from build123d import *

# Parameters (mm, degrees)
SKETCH1_R           = 2.1
SKETCH1_R_2         = 3.4
BOSS_EXTRUDE1_DEPTH = 160


with BuildPart() as part:
    # Sketch1 → Boss-Extrude1 (new body)
    with BuildSketch(Plane(origin=(0, 0, 0), x_dir=(0, 0, -1), z_dir=(1, 0, 0))):
        with BuildLine():
            Line((-15, 28), (-15, 19))
            Line((-15, 19), (-13, 19))
            Line((-13, 19), (-13, 23.25))
            Line((-13, 23.25), (-9.664213562, 23.25))
            Line((-9.664213562, 23.25), (-6, 19.585786438))
            Line((-6, 19.585786438), (-6, 10.414213562))
            Line((-6, 10.414213562), (-9.664213562, 6.75))
            Line((-9.664213562, 6.75), (-13, 6.75))
            Line((-13, 6.75), (-13, 11))
            Line((-13, 11), (-15, 11))
            Line((-15, 11), (-15, -11))
            Line((-15, -11), (-13, -11))
            Line((-13, -11), (-13, -6.75))
            Line((-13, -6.75), (-9.664213562, -6.75))
            Line((-9.664213562, -6.75), (-6, -10.414213562))
            Line((-6, -10.414213562), (-6, -19.585786438))
            Line((-6, -19.585786438), (-9.664213562, -23.25))
            Line((-9.664213562, -23.25), (-13, -23.25))
            Line((-13, -23.25), (-13, -19))
            Line((-13, -19), (-15, -19))
            Line((-15, -19), (-15, -28))
            ThreePointArc((-15, -28), (-14.414213562, -29.414213562), (-13, -30))
            Line((-13, -30), (-4, -30))
            Line((-4, -30), (-4, -28))
            Line((-4, -28), (-8.25, -28))
            Line((-8.25, -28), (-8.25, -24.664213562))
            Line((-8.25, -24.664213562), (-4.585786438, -21))
            Line((-4.585786438, -21), (4.585786438, -21))
            Line((4.585786438, -21), (8.25, -24.664213562))
            Line((8.25, -24.664213562), (8.25, -28))
            Line((8.25, -28), (4, -28))
            Line((4, -28), (4, -30))
            Line((4, -30), (13, -30))
            ThreePointArc((13, -30), (14.414213562, -29.414213562), (15, -28))
            Line((15, -28), (15, -19))
            Line((15, -19), (13, -19))
            Line((13, -19), (13, -23.25))
            Line((13, -23.25), (9.664213562, -23.25))
            Line((9.664213562, -23.25), (6, -19.585786438))
            Line((6, -19.585786438), (6, -10.414213562))
            Line((6, -10.414213562), (9.664213562, -6.75))
            Line((9.664213562, -6.75), (13, -6.75))
            Line((13, -6.75), (13, -11))
            Line((13, -11), (15, -11))
            Line((15, -11), (15, 11))
            Line((15, 11), (13, 11))
            Line((13, 11), (13, 6.75))
            Line((13, 6.75), (9.664213562, 6.75))
            Line((9.664213562, 6.75), (6, 10.414213562))
            Line((6, 10.414213562), (6, 19.585786438))
            Line((6, 19.585786438), (9.664213562, 23.25))
            Line((9.664213562, 23.25), (13, 23.25))
            Line((13, 23.25), (13, 19))
            Line((13, 19), (15, 19))
            Line((15, 19), (15, 28))
            ThreePointArc((15, 28), (14.414213562, 29.414213562), (13, 30))
            Line((13, 30), (4, 30))
            Line((4, 30), (4, 28))
            Line((4, 28), (8.25, 28))
            Line((8.25, 28), (8.25, 24.664213562))
            Line((8.25, 24.664213562), (4.585786438, 21))
            Line((4.585786438, 21), (-4.585786438, 21))
            Line((-4.585786438, 21), (-8.25, 24.664213562))
            Line((-8.25, 24.664213562), (-8.25, 28))
            Line((-8.25, 28), (-4, 28))
            Line((-4, 28), (-4, 30))
            Line((-4, 30), (-13, 30))
            ThreePointArc((-13, 30), (-14.414213562, 29.414213562), (-15, 28))
        make_face()
        with Locations((-11.6, 26.625)):
            Circle(SKETCH1_R, mode=Mode.SUBTRACT)
        with Locations((0, 15)):
            Circle(SKETCH1_R_2, mode=Mode.SUBTRACT)
        with Locations((11.6, 26.625)):
            Circle(SKETCH1_R, mode=Mode.SUBTRACT)
        with Locations((0, -15)):
            Circle(SKETCH1_R_2, mode=Mode.SUBTRACT)
        with Locations((-11.6, -26.625)):
            Circle(SKETCH1_R, mode=Mode.SUBTRACT)
        with Locations((11.6, -26.625)):
            Circle(SKETCH1_R, mode=Mode.SUBTRACT)
        with BuildLine():
            Line((-8.835786438, 4.75), (-12, 4.75))
            ThreePointArc((-12, 4.75), (-12.707106781, 4.457106781), (-13, 3.75))
            Line((-13, 3.75), (-13, -3.75))
            ThreePointArc((-13, -3.75), (-12.707106781, -4.457106781), (-12, -4.75))
            Line((-12, -4.75), (-8.835786438, -4.75))
            Line((-8.835786438, -4.75), (-3.651792162, -9.933994275))
            ThreePointArc((-3.651792162, -9.933994275), (-3.470780401, -10.020243756), (-3.275866789, -9.973202134))
            ThreePointArc((-3.275866789, -9.973202134), (0, -9), (3.275866789, -9.973202134))
            ThreePointArc((3.275866789, -9.973202134), (3.470780401, -10.020243756), (3.651792162, -9.933994275))
            Line((3.651792162, -9.933994275), (8.835786438, -4.75))
            Line((8.835786438, -4.75), (12, -4.75))
            ThreePointArc((12, -4.75), (12.707106781, -4.457106781), (13, -3.75))
            Line((13, -3.75), (13, 3.75))
            ThreePointArc((13, 3.75), (12.707106781, 4.457106781), (12, 4.75))
            Line((12, 4.75), (8.835786438, 4.75))
            Line((8.835786438, 4.75), (3.651792162, 9.933994275))
            ThreePointArc((3.651792162, 9.933994275), (3.470780401, 10.020243756), (3.275866789, 9.973202134))
            ThreePointArc((3.275866789, 9.973202134), (0, 9), (-3.275866789, 9.973202134))
            ThreePointArc((-3.275866789, 9.973202134), (-3.470780401, 10.020243756), (-3.651792162, 9.933994275))
            Line((-3.651792162, 9.933994275), (-8.835786438, 4.75))
        make_face(mode=Mode.SUBTRACT)
    extrude(amount=BOSS_EXTRUDE1_DEPTH)


solid = part.part
Design review of the part built by this model. Coordinates are the model's own, in mm. Give positions to 0.01 mm unless a question says otherwise; leave off trailing zeros. Loops run counter-clockwise (first coordinate to the right, second up) from the corner with the lowest first, then second, coordinate; pieces in that order, holes last. Notation, with made-up numbers: (75.25, 86.5) - (112.25, 86.5) arc R10 ccw to (112.25, 104.5) - close; hole circle Ø4 at (87.5, 61.5). An arc over 180 degrees is marked (long way). Write item = value, one per line.
1) Take a section at D-D on x = 79.5. Count the separate pieces of the cut face and the enclosed holes in it, and give its area (4 significant figures).
Result sheet:
separate_pieces = 1
enclosed_holes = 7
area = 592.5 mm2
2) Take a section at A-A on y = 2. State the section outline as (x, z) points, and give its area (3 significant figures).
Result sheet:
outline = (0, -15) - (160, -15) - (160, -13) - (0, -13) - close; (0, 13) - (160, 13) - (160, 15) - (0, 15) - close
area = 640 mm2
3) Take a section at B-B on z = 0. State the section outline as (x, y) points, and give its area (3 significant figures).
Result sheet:
outline = (0, -21) - (160, -21) - (160, -18.4) - (0, -18.4) - close; (0, -11.6) - (160, -11.6) - (160, -9) - (0, -9) - close; (0, 9) - (160, 9) - (160, 11.6) - (0, 11.6) - close; (0, 18.4) - (160, 18.4) - (160, 21) - (0, 21) - close
area = 1,660 mm2
4) Take a section at C-C on y = -15. State the section outline as (x, z) points, and give its area (3 significant figures).
Result sheet:
outline = (0, -6) - (160, -6) - (160, -3.4) - (0, -3.4) - close; (0, 3.4) - (160, 3.4) - (160, 6) - (0, 6) - close
area = 832 mm2
5) Draft analysis for pull direction Y (two halves, no side actions). For faces 1 (the face through (79, -28, -6)), 2 (the face through (79, -30, -8)), 3 (the face through (79, -24, -15)), state which applies: +Y half, -Y half, draft (parallel to the pull), parting line (faces both ways), or undercut.
Result sheet:
face_1 = undercut
face_2 = -Y half
face_3 = draft
6) To check wall thickness, follow line 1 (Y direction, x = 84, z = 0); line 2 (Y direction, x = 122, z = -11.6) (3 decimals); line 3 (Z direction, x = 68.5, y = 1.5). State the ranges of each line that lie inside material, in increasing order.
Result sheet:
line_1 = -21 to -18.4, -11.6 to -9, 9 to 11.6, 18.4 to 21
line_2 = -30 to -28.725, -24.525 to -23.25, -6.75 to -4.75, 4.75 to 6.75, 23.25 to 24.525, 28.725 to 30
line_3 = -15 to -13, 13 to 15
7) Clearance check with flat-ended pins moving along their axes: pin 1 Ø2 at (x, z) = (71, 14) entering from +Y; pin 2 Ø2 at (x, y) = (113, 29.5) entering from -Z; pin 3 Ø3 at (x, y) = (119.5, 13.5) entering from -Z. State where each tip first meets the part, or that it passes through.
Result sheet:
pin_1 = 30
pin_2 = -14.94
pin_3 = -6
